Can you work these out from the model? Positions are in its coordinate system, mm. Face numbers are marked on the shaded views. A direction names the side the tool comes from. Round coordinates to 2 decimals unless told otherwise and drop trailing zeros.
(1) I want a section at A-A on z = 0. Give the number of separate pieces and of enclosed holes in the cut face, plus the area to 3 significant figures.
(2) Will these pins go through, and if not, where does the flat tip stop? pin 1 Ø0.8 at (x, z) = (4.95, 4.95) entering from -Y; pin 2 Ø4 at (x, z) = (3, 6.5) entering from +Y; pin 3 Ø1.6 at (x, z) = (0, -7) entering from -Y; pin 4 Ø1 at (y, z) = (3, -1.5) entering from -X.
(3) Which directions (+Z, -Z, +X, -X, +Y, -Y) give clear straight access to the entire face, cutting with the end or side of a thin tool? Please do the marked faces 5 and 6.
(4) If I drill on line 1 along X through (y, z) = (1, 3.5); line 2 along X through (y, z) = (0.95, -5); line 3 along Z through (x, y) = (2.75, 2), over which ranges is the centre line in solid material (lowest first)?
(5) Thinking about a two-plate mould opening in Z: for the marked faces 1, 2, 3 and 4, which applies, released by +Z, released by -Z, zero draft, split by the parting line, or undercut?
from build123d import *

# Parameters (mm, degrees)
SKETCH1_R                = 9.8
SKETCH1_R_2              = 0.685
SKETCH1_R_3              = 1.525
BOSS_EXTRUDE1_DEPTH      = 4.25
SHELL3_T                 = -1.2
BOSS_EXTRUDE2_DEPTH      = 0.5
BOSS_EXTRUDE2_DEPTH_BACK = 4.25
SKETCH2_R                = 4.4
SKETCH2_R_2              = 1.525
SKETCH3_R                = 2.5
CUT_EXTRUDE1_DEPTH       = 3.15
SKETCH4_R                = 3.75
SKETCH4_R_2              = 1.525
BOSS_EXTRUDE3_DEPTH      = 0.25
FILLET1_R                = 0.1


with BuildPart() as part:
    # Sketch1 → Boss-Extrude1 (new body)
    with BuildSketch(Plane(origin=(0, 0, 0), x_dir=(1, 0, 0), z_dir=(0, 1, 0))):
        with Locations(Location((0, 0, 0), (0, 0, 270))):
            Circle(SKETCH1_R)
        with Locations(Location((0, 7, 0), (0, 0, 270))):
            Circle(SKETCH1_R_2, mode=Mode.SUBTRACT)
        with Locations(Location((4.949747468, 4.949747468, 0), (0, 0, 270))):
            Circle(SKETCH1_R_2, mode=Mode.SUBTRACT)
        with Locations(Location((7, 0, 0), (0, 0, 270))):
            Circle(SKETCH1_R_2, mode=Mode.SUBTRACT)
        with Locations(Location((4.949747468, -4.949747468, 0), (0, 0, 270))):
            Circle(SKETCH1_R_2, mode=Mode.SUBTRACT)
        with Locations(Location((0, -7, 0), (0, 0, 270))):
            Circle(SKETCH1_R_2, mode=Mode.SUBTRACT)
        with Locations(Location((-4.949747468, -4.949747468, 0), (0, 0, 270))):
            Circle(SKETCH1_R_2, mode=Mode.SUBTRACT)
        with Locations(Location((-7, 0, 0), (0, 0, 270))):
            Circle(SKETCH1_R_2, mode=Mode.SUBTRACT)
        with Locations(Location((-4.949747468, 4.949747468, 0), (0, 0, 270))):
            Circle(SKETCH1_R_2, mode=Mode.SUBTRACT)
        with Locations(Location((0, 0, 0), (0, 0, 270))):
            Circle(SKETCH1_R_3, mode=Mode.SUBTRACT)
    extrude(amount=BOSS_EXTRUDE1_DEPTH)

    # Shell3
    shell3_openings = [part.faces().sort_by_distance(p)[0] for p in [
        (0, 0, -9.522814142),
    ]]
    offset(amount=SHELL3_T, openings=shell3_openings)

    # Sketch2 → Boss-Extrude2 (add, two sides: drawn at the far end of the back side and taken through both)
    with BuildSketch(Plane.XZ.offset(-BOSS_EXTRUDE2_DEPTH_BACK)):
        with Locations(Location((0, 0, 0), (0, 0, 270))):
            Circle(SKETCH2_R)
        with Locations(Location((0, 0, 0), (0, 0, 270))):
            Circle(SKETCH2_R_2, mode=Mode.SUBTRACT)
    extrude(amount=BOSS_EXTRUDE2_DEPTH + BOSS_EXTRUDE2_DEPTH_BACK)

    # Sketch3 → Cut-Extrude1 (cut)
    with BuildSketch(Plane.XZ.offset(0.5)):
        with Locations(Location((0, 0, 0), (0, 0, 270))):
            Circle(SKETCH3_R)
    extrude(amount=-CUT_EXTRUDE1_DEPTH, mode=Mode.SUBTRACT)

    # Sketch4 → Boss-Extrude3 (add)
    with BuildSketch(Plane(origin=(0, 4.25, 0), x_dir=(1, 0, 0), z_dir=(0, 1, 0))):
        with Locations(Location((0, 0, 0), (0, 0, 270))):
            Circle(SKETCH4_R)
        with Locations(Location((0, 0, 0), (0, 0, 90))):
            Circle(SKETCH4_R_2, mode=Mode.SUBTRACT)
    extrude(amount=BOSS_EXTRUDE3_DEPTH)

    # Fillet1
    fillet1_edges = [part.edges().sort_by_distance(p)[0] for p in [
        (0, 4.25, -3.75),
    ]]
    fillet(fillet1_edges, radius=FILLET1_R)


solid = part.part
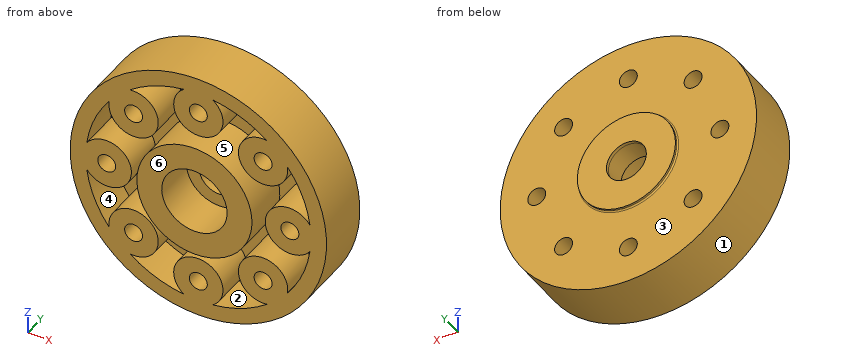
Filled sheet:
1. separate pieces: 4
1. enclosed holes: 0
1. area: 52.2 mm2
2. pin 1: passes through
2. pin 2: stops at y = 4.25
2. pin 3: stops at y = 0
2. pin 4: stops at x = -9.75
3. face 5: -Y
3. face 6: +Z, -Z, +X, -X, -Y
4. line 1: x = -9.15 to -7.86, -6.15 to -3.74, -2.67 to 2.67, 3.74 to 6.15, 7.86 to 9.15
4. line 2: x = -8.43 to -7, -6.83 to -5.63, -4.27 to -3.07, 3.07 to 4.27, 5.63 to 6.83, 7 to 8.43
4. line 3: z = -9.41 to -8.15, -3.43 to 3.43, 8.15 to 9.41
5. face 1: split by the parting line
5. face 2: undercut
5. face 3: zero draft
5. face 4: undercut
